Autodesk Inventor part; units mm, degrees
ref_plane "YZ Plane" through (0, 0, 0) normal (1, 0, 0) x (0, 1, 0)
ref_plane "XZ Plane" through (0, 0, 0) normal (0, 1, 0) x (-1, 0, 0)
ref_plane "XY Plane" through (0, 0, 0) normal (0, 0, 1) x (1, 0, 0)
sketch "Szkic1" plane through (0, 0, 0) normal (0, 0, 1) x (1, 0, 0)
  line L0 (54, -15.2042) -> (54, -5)
  line L1 (18, -31) -> (52, -31)
  circle A0 centre (35, -25.5) radius 3.5
  circle A1 centre (26, -7) radius 3.5
  circle A2 centre (44, -7) radius 3.5
  line L2 (18, -31) -> (52, -31)
  line L3 (54, -24.7958) -> (54, -29)
  line L4 (54, -15.2042) -> (54, -5)
  line L5 (52, -3) -> (18, -3)
  line L6 (16, -5) -> (16, -15.2042)
  line L7 (16, -24.7958) -> (16, -20)
  line L8 (85, -3) -> (85, 41.8489)
  line L9 (-15, 44.8489) -> (85, 44.8489)
  line L10 (-15, -3) -> (-15, 41.8489)
  line L11 (-15, -4) -> (15.8, -4)
  line L12 (85, 44.8489) -> (-15, 44.8489)
  line L13 (-15, 44.8489) -> (-15, -3)
  line L14 (-15, -3) -> (85, -3)
  line L15 (85, -3) -> (85, 44.8489)
  line L16 (52, -31) -> (16, -31)
  line L17 (16, -31) -> (16, -3)
  line L18 (16, -3) -> (52, -3)
  line L19 (52, -3) -> (52, -31)
  arc A3 (54, -5) -> (52, -3) centre (52, -5) ccw
  arc A4 (18, -3) -> (16, -5) centre (18, -5) ccw
  line L20 (16, -15.2042) -> (16, -20)
  line L21 (16, -29) -> (16, -24.7958)
  arc A5 (16, -29) -> (18, -31) centre (18, -29) ccw
  arc A6 (52, -31) -> (54, -29) centre (52, -29) ccw
  line L22 (54, -15.2042) -> (54, -24.7958)
  line L23 (54, -15.2042) -> (54, -15.2042)
  point P0 (0, 0)
  point P1 (54, -3)
  point P2 (52, -3)
extrude "Wyciągnięcie proste1" add sketch "Szkic1" along normal blind 2 contours L5 L14 L10 L13 L9 L15 L8
sketch "Szkic2" plane through (0, 0, 2) normal (0, 0, 1) x (1, 0, 0)
  circle A0 centre (81.5, 0.5) radius 2
  circle A1 centre (81.5, 28.3844) radius 2
  circle A2 centre (-11.5, 28.3844) radius 2
  circle A3 centre (-11.5, 0.5) radius 2
  point P0 (0, 0)
hole "Otwór1" at (81.5, 0.5, 2) at (81.5, 28.3844, 2) at (-11.5, 0.5, 2) at (-11.5, 28.3844, 2) direction (0, 0, -1) diameter 3.2 depth 7 tip angle 118 countersink diameter 3.8 countersink angle 90
sketch "Szkic3" plane through (0, 0, 2) normal (0, 0, 1) x (1, 0, 0)
  circle A0 centre (35, -25.5) radius 3.5
  circle A1 centre (26, -7) radius 3.5
  circle A2 centre (44, -7) radius 3.5
  arc A3 (54, -5) -> (52, -3) centre (52, -5) ccw
  line L0 (52, -3) -> (18, -3)
  arc A4 (18, -3) -> (16, -5) centre (18, -5) ccw
  line L1 (16, -5) -> (16, -15.2042)
  line L2 (16, -15.2042) -> (16, -20)
  line L3 (16, -24.7958) -> (16, -20)
  line L4 (16, -29) -> (16, -24.7958)
  arc A5 (16, -29) -> (18, -31) centre (18, -29) ccw
  line L5 (18, -31) -> (52, -31)
  arc A6 (52, -31) -> (54, -29) centre (52, -29) ccw
  line L6 (54, -24.7958) -> (54, -29)
  line L7 (54, -20) -> (54, -24.7958)
  line L8 (54, -20) -> (54, -15.2042)
  line L9 (54, -15.2042) -> (54, -5)
  circle A7 centre (-11.5, 0.5) radius 1.9
  circle A8 centre (81.5, 0.5) radius 1.9
  circle A9 centre (81.5, 28.3844) radius 1.9
  circle A10 centre (-11.5, 28.3844) radius 1.9
  line L10 (85, 44.8489) -> (-15, 44.8489)
  line L11 (-15, 44.8489) -> (-15, -3)
  line L12 (-15, -3) -> (85, -3)
  line L13 (85, -3) -> (85, 44.8489)
  line L14 (16, -5) -> (16, -3)
  line L15 (54, -5) -> (54, -3)
  point P0 (0, 0)
  point P1 (52, -3)
extrude "Wyciągnięcie proste2" add sketch "Szkic3" against normal up to surface (2 mm away) contours A0 | A1 | A2 | L9 L8 L7 L6 A6 L5 A5 L4 L3 L2 L1 A4 L0 A3 | A3 L12 L15 | A4 L14 L12
fillet "Zaokrąglenie1" radius 2 6 edges at (85, -3, 1) (54, -3, 1) (85, 44.8489, 1) (16, -3, 1) (-15, -3, 1) (-15, 44.8489, 1)
properties part number "pokrywa"
Verification items for the finished model (mm, model axes). A direction names the side the tool comes from. Coordinates: 2 decimals unless noted, no trailing zeros. Order: outer loops, then holes, each group sorted by start corner. A loop starts at its lowest first (then second) coordinate and runs counter-clockwise, first axis right, second up.
1. Release check for a two-part mould opening along Y. For faces 4 (the face through (16, -17, 1)), 5 (the face through (-13.086, 0.708, 0.838)), 6 (the face through (-14.43, -2.4, 1.01)) record: +Y half, -Y half, draft (parallel to the pull), parting line (faces both ways), or undercut.
Results found:
face 4: draft
face 5: undercut
face 6: -Y half
2. Sectioned sample at D-D, the plane x = 72. Record the cut outline in (y, z).
Results found:
outline: (-3, 0) - (44.85, 0) - (44.85, 2) - (-3, 2) - close
3. Sectioned sample at B-B, the plane x = -11.5. Record the cut outline in (y, z), and give its area (3 significant figures).
Results found:
outline: (-3, 0) - (-1.1, 0) - (-1.1, 1.7) - (-1.4, 2) - (-3, 2) - close; (2.1, 0) - (26.78, 0) - (26.78, 1.7) - (26.48, 2) - (2.4, 2) - (2.1, 1.7) - close; (29.98, 0) - (44.85, 0) - (44.85, 2) - (30.28, 2) - (29.98, 1.7) - close
area: 82.7 mm2
4. Go/stop test with flat-tipped pins: pin 1 Ø2.5 at (x, y) = (81.5, 28.38) entering from +Z; pin 2 Ø0.6 at (x, z) = (-4.5, 1) entering from -Y; pin 3 Ø1 at (y, z) = (-4, 1.5) entering from +X. Record where each tip stops, or that it passes through.
Results found:
pin 1: passes through
pin 2: stops at y = -3
pin 3: stops at x = 54.68
5. Sectioned sample at C-C, the plane z = 0.75. Record the cut outline in (x, y).
Results found:
outline: (-15, -1) arc R2 ccw to (-13, -3) - (14, -3) arc R2 cw to (16, -5) - (16, -29) arc R2 ccw to (18, -31) - (52, -31) arc R2 ccw to (54, -29) - (54, -5) arc R2 cw to (56, -3) - (83, -3) arc R2 ccw to (85, -1) - (85, 42.85) arc R2 ccw to (83, 44.85) - (-13, 44.85) arc R2 ccw to (-15, 42.85) - close; hole circle Ø3.2 at (-11.5, 0.5); hole circle Ø3.2 at (-11.5, 28.38); hole circle Ø3.2 at (81.5, 0.5); hole circle Ø3.2 at (81.5, 28.38)
6. Scan lines: line 1 (Y direction, x = 81.5, z = 0.75); line 2 (X direction, y = 0.5, z = 0.8); line 3 (Y direction, x = 12, z = 1.6). Record each from-to range of solid material in increasing order.
Results found:
line 1: y = -3 to -1.1, 2.1 to 26.78, 29.98 to 44.85
line 2: x = -15 to -13.1, -9.9 to 79.9, 83.1 to 85
line 3: y = -3 to 44.85
7. Sectioned sample at A-A, the plane y = 0.5. Record the cut outline in (x, z), and give its area (3 significant figures).
Results found:
outline: (-15, 0) - (-13.1, 0) - (-13.1, 1.7) - (-13.4, 2) - (-15, 2) - close; (-9.9, 0) - (79.9, 0) - (79.9, 1.7) - (79.6, 2) - (-9.6, 2) - (-9.9, 1.7) - close; (83.1, 0) - (85, 0) - (85, 2) - (83.4, 2) - (83.1, 1.7) - close
area: 187 mm2
8. Set-up check for faces 1 (the face through (1, -3, 1)), 2 (the face through (-15, 21, 1)), 3 (the face through (70, -3, 1)): record each of +Z, -Z, +X, -X, +Y, -Y from which the full face is reachable in a straight line by a thin tool's end or side.
Results found:
face 1: +Z, -Z, -X, -Y
face 2: +Z, -Z, -X, +Y, -Y
face 3: +Z, -Z, +X, -Y
